from build123d import *

# Parameters (mm, degrees)
SKETCH1_R           = 6.35
BOSS_EXTRUDE1_DEPTH = 6.35
BOSS_EXTRUDE1_TAPER = 15
SKETCH2_R           = 3.175
CUT_EXTRUDE1_DEPTH  = 3.96875
SKETCH3_R           = 1.5875
CUT_EXTRUDE2_DEPTH  = 3.38125


with BuildPart() as part:
    # Sketch1 → Boss-Extrude1 (new body)
    with BuildSketch(Plane.XY):
        Circle(SKETCH1_R)
    extrude(amount=BOSS_EXTRUDE1_DEPTH, taper=BOSS_EXTRUDE1_TAPER)

    # Sketch2 → Cut-Extrude1 (cut)
    with BuildSketch(Plane.XY.offset(6.35)):
        Circle(SKETCH2_R)
    extrude(amount=-CUT_EXTRUDE1_DEPTH, mode=Mode.SUBTRACT)

    # Sketch3 → Cut-Extrude2 (cut, through all)
    with BuildSketch(Plane.XY.offset(2.38125)):
        Circle(SKETCH3_R)
    extrude(amount=-CUT_EXTRUDE2_DEPTH, mode=Mode.SUBTRACT)


solid = part.part
Can you work these out from the model? Positions are in its coordinate system, mm. A direction names the side the tool comes from. Coordinates: 2 decimals unless noted, no trailing zeros. Order: outer loops, then holes, each group sorted by start corner. A loop starts at its lowest first (then second) coordinate and runs counter-clockwise, first axis right, second up. Notation, with made-up numbers: (5, -15.75) -> (41, -15.75) arc R28 ccw to (41, 7.25) -> close; hole circle Ø6 at (28, 37.5). An arc over 180 degrees is marked (long way). Use one line per item in the form item = value.
Q1. Imagine slicing it at C-C, the plane z = 0.75. List the corners of the cut face in (x, y) for me (1 decimal), then the cut area to 3 significant figures.
From the geometry:
outline = circle Ø12.3 at (0, 0); hole circle Ø3.2 at (0, 0)
area = 111 mm²
Q2. Which directions (+Z, -Z, +X, -X, +Y, -Y) give clear straight access to the entire face, cutting with the end or side of a thin tool? Please do faces 1 (the face through (-0.34, -1.55, 1.21)), 2 (the face through (-0.69, -3.1, 4.39)).
From the geometry:
face_1 = +Z, -Z
face_2 = +Z
Q3. I need wall thicknesses on L1, parallel to Y at x = 0, z = 3.8 (3 decimals); L2, parallel to Y at x = -2.75, z = 5.25; L3, parallel to X at y = -1.5, z = 3.5. Which ranges of each line are inside material? Lowest first, please.
From the geometry:
L1 = -5.332 to -3.175, 3.175 to 5.332
L2 = -4.11 to -1.59, 1.59 to 4.11
L3 = -5.2 to -2.8, 2.8 to 5.2
Q4. We'd pull the mould along X, two halves only. Please class faces 3 (the face through (1.4, -1.4, 2.381)), 4 (the face through (1.3, -1.3, 0)), 5 (the face through (-4.055, -3.109, 4.631)): released by +X, released by -X, zero draft, split by the parting line, or undercut.
From the geometry:
face_3 = undercut
face_4 = zero draft
face_5 = split by the parting line
Q5. Will these pins go through, and if not, where does the flat tip stop? P1, Ø2, axis at y = -0.5, z = 4, coming from the +X side; P2, Ø5, axis at x = 0, y = 0, coming from the -Z side; P3, Ø1, axis at x = 3.5, z = 4.5, coming from the +Y side.
From the geometry:
P1 = 5.53
P2 = 0
P3 = 4.21
Q6. Imagine slicing it at D-D, the plane z = 2.75. List the corners of the cut face in (x, y) for me (3 decimals).
From the geometry:
outline = circle Ø11.226 at (0, 0); hole circle Ø6.35 at (0, 0)
